Source: CAD feature listing. Evaluate the final solid. Frame: model axes, mm. Face numbers are marked on the shaded views. A direction names the side the tool comes from. Coordinates: 2 decimals unless noted, no trailing zeros. Write each loop counter-clockwise with the first axis right and the second up, starting at its lowest first coordinate (ties: lowest second). Pieces come first, ordered by that corner, then holes. Notation, with made-up numbers: M -7,4.5 L 35,4.5 A18 ccw 35,16.5 Z; hole C -10.75,-22.75 d4. An arc over 180 degrees is marked long. Answer as CSV lines item,"result". Start each with the question number.
1. Line query: probe 1 along Z at (x, y) = (31, 60.5); probe 2 along Z at (x, y) = (-30, 22); probe 3 along Z at (x, y) = (20.5, 15). Output: solid intervals per line, ascending. Write a range as [from, to].
2. Section B-B on x = 17. Return the cut outline in (y, z), plus the area to 3 significant figures.
3. Contact query for flat-ended pins moving along their axis: pin 1 Ø8 at (x, y) = (43.5, 59.5) entering from +Z; pin 2 Ø5.5 at (x, z) = (-6, -89) entering from -Y; pin 3 Ø6 at (y, z) = (49, -78) entering from +X; pin 4 Ø5.5 at (x, y) = (45.99, 41.5) entering from -Z. Output: stop coordinate, or through.
4. Mould query, pull axis Z, two halves, no side actions, for the marked faces 1 and 2. Classes: pulls with the +Z half, pulls with the -Z half, needs draft (parallel to the pull), parting line crosses it, or undercut.
5. Section A-A on x = 0. Return the cut outline in (y, z).
6. Reachability of the marked faces 3 and 4 from +Z, -Z, +X, -X, +Y, -Y: full face, straight path, thin tool, end or side. Return the list, or none.
```python
from build123d import *

# Parameters (mm, degrees)
SKETCH9_R      = 2.928820999
EXTRUDE2_DEPTH = 7.62
FILLET3_R      = 2.54


with BuildPart() as part:
    # Sweep5: sweep along a path in Sketch1
    with BuildLine(Plane(origin=(0, 0, 0), x_dir=(0, 0, -1), z_dir=(1, 0, 0))) as sweep5_path:
        Line((0, 0), (65.991135768, 38.1))
        ThreePointArc((65.991135768, 38.1), (72.117132023, 40.637470732), (78.691135768, 41.502954744))
        Line((78.691135768, 41.502954744), (90.878802907, 41.502954744))
    # Sketch2 → Sweep5 (sweep)
    with BuildSketch(Plane(origin=(0, 0, 0), x_dir=(-1, 0, 0), z_dir=(0, 0.5000000000000013, -0.8660254037844379))):
        with BuildLine():
            Line((-25.4, 12.7), (25.4, 12.7))
            ThreePointArc((25.4, 12.7), (38.1, 0), (25.4, -12.7))
            Line((25.4, -12.7), (-25.4, -12.7))
            ThreePointArc((-25.4, -12.7), (-38.1, 0), (-25.4, 12.7))
        make_face()
    sweep(path=sweep5_path.line)

    # Sketch9 → Extrude2 (add)
    with BuildSketch(Plane(origin=(0, 0, -90.878802907), x_dir=(-1, 0, 0), z_dir=(0, 0, -1))):
        with BuildLine():
            Line((-25.4, 70.712954744), (25.4, 70.712954744))
            ThreePointArc((25.4, 70.712954744), (54.61, 41.502954744), (25.4, 12.292954744))
            Line((25.4, 12.292954744), (-25.4, 12.292954744))
            ThreePointArc((-25.4, 12.292954744), (-54.61, 41.502954744), (-25.4, 70.712954744))
        make_face()
        with Locations(Location((-45.990959388, 41.502954744, 0), (0, 0, 90))):
            Circle(SKETCH9_R, mode=Mode.SUBTRACT)
        with Locations(Location((0, 62.457954744, 0), (0, 0, 90))):
            Circle(SKETCH9_R, mode=Mode.SUBTRACT)
        with Locations(Location((46.355, 41.502954744, 0), (0, 0, 90))):
            Circle(SKETCH9_R, mode=Mode.SUBTRACT)
        with Locations(Location((0, 20.547954744, 0), (0, 0, 90))):
            Circle(SKETCH9_R, mode=Mode.SUBTRACT)
        with BuildLine():
            Line((-25.4, 54.202954744), (25.4, 54.202954744))
            ThreePointArc((25.4, 54.202954744), (38.1, 41.502954744), (25.4, 28.802954744))
            Line((25.4, 28.802954744), (-25.4, 28.802954744))
            ThreePointArc((-25.4, 28.802954744), (-38.1, 41.502954744), (-25.4, 54.202954744))
        make_face(mode=Mode.SUBTRACT)
    extrude(amount=-EXTRUDE2_DEPTH)

    # Fillet3
    fillet3_edges = [part.edges().sort_by_distance(p)[0] for p in [
        (54.61, 41.502954744, -83.258802907),
        (0, 70.712954744, -83.258802907),
        (-54.61, 41.502954744, -83.258802907),
        (0, 12.292954744, -83.258802907),
        (38.1, 41.502954744, -83.258802907),
        (0, 28.802954744, -83.258802907),
        (-38.1, 41.502954744, -83.258802907),
        (0, 54.202954744, -83.258802907),
    ]]
    fillet(fillet3_edges, radius=FILLET3_R)


solid = part.part
```
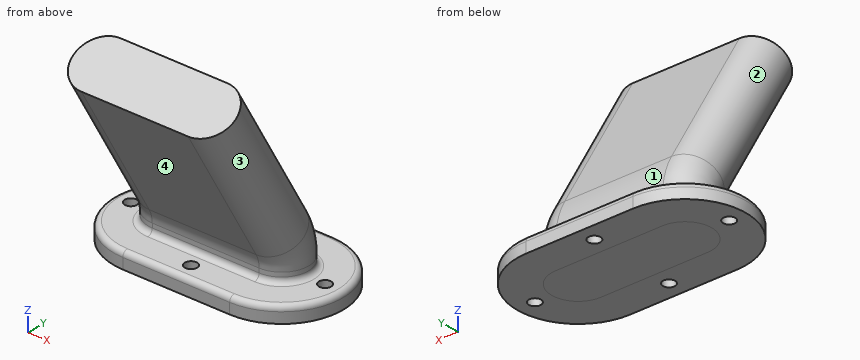
Values:
1,probe 1,"[-90.88, -83.26]"
1,probe 2,"[-90.88, -83.26], [-61.78, -14.43]"
1,probe 3,"[-90.88, -83.26], [-51.38, -0.58]"
2,outline,"M -11,-6.35 L 27.1,-72.34 A12.7 cw 28.8,-78.69 L 28.8,-80.72 A2.54 cw 26.26,-83.26 L 14.83,-83.26 A2.54 ccw 12.29,-85.8 L 12.29,-90.88 L 70.71,-90.88 L 70.71,-85.8 A2.54 ccw 68.17,-83.26 L 56.74,-83.26 A2.54 cw 54.2,-80.72 L 54.2,-78.69 A38.1 ccw 49.1,-59.64 L 11,6.35 Z"
2,area,"2,830 mm²"
3,pin 1,"z = -83.26"
3,pin 2,"y = 12.29"
3,pin 3,"x = 37.27"
3,pin 4,"through"
4,face 1,"pulls with the +Z half"
4,face 2,"undercut"
5,outline,"M -11,-6.35 L 27.1,-72.34 A12.7 cw 28.8,-78.69 L 28.8,-80.72 A2.54 cw 26.26,-83.26 L 23.48,-83.26 L 23.48,-90.88 L 59.53,-90.88 L 59.53,-83.26 L 56.74,-83.26 A2.54 cw 54.2,-80.72 L 54.2,-78.69 A38.1 ccw 49.1,-59.64 L 11,6.35 Z; M 12.29,-90.88 L 17.62,-90.88 L 17.62,-83.26 L 14.83,-83.26 A2.54 ccw 12.29,-85.8 Z; M 65.39,-90.88 L 70.71,-90.88 L 70.71,-85.8 A2.54 ccw 68.17,-83.26 L 65.39,-83.26 Z"
6,face 3,"+X"
6,face 4,"+X, -X, -Y"
